Build history of the part. All positions in model axes, mm. A direction names the side the tool comes from. Round coordinates to 2 decimals unless told otherwise and drop trailing zeros. Loops run counter-clockwise (first coordinate to the right, second up) from the corner with the lowest first, then second, coordinate; pieces in that order, holes last. Notation, with made-up numbers: (-7.75, 63.5) - (44.25, 63.5) arc R19 ccw to (44.25, 84.5) - close; hole circle Ø8 at (59.5, 40). An arc over 180 degrees is marked (long way). Put each result on its own line as item: value. Start each with the question number.
from build123d import *

# Parameters (mm, degrees)
F1_DEPTH = 12


# Not quite as in the source:
# - a feature names something its author has since deleted; it is built from what else it names


with BuildPart() as f1:
    # F0 (on Front) → F1 (new body)
    with BuildSketch(Plane.XZ):
        with BuildLine():
            Line((-78.3512531443, 52.5226152241), (-78.3512531443, -23.4773847759))
            Line((-78.3512531443, -23.4773847759), (48.6487468557, -23.4773847759))
            Line((48.6487468557, -23.4773847759), (163.7198627451, -39.3522962011))
            ThreePointArc((163.7198627451, -39.3522962011), (169.4031778605, -34.3992082296), (163.7198627451, -29.4461202581))
            ThreePointArc((163.7198627451, -29.4461202581), (140.2372169997, 8.5604113595), (135.6487468557, 53))
            Line((135.6487468557, 53), (129.9201593475, 53))
            Line((129.9201593475, 53), (-55.8512531443, 53))
            Line((-55.8512531443, 53), (-78.3512531443, 53))
            Line((-78.3512531443, 53), (-78.3512531443, 52.5226152241))
        make_face()
        with BuildLine():
            Line((-63.3512531443, 7.5), (-63.3512531443, 21.5))
            Line((-63.3512531443, 21.5), (-63.3512531443, 35.5))
            ThreePointArc((-63.3512531443, 35.5), (-55.8512531443, 43), (-48.3512531443, 35.5))
            Line((-48.3512531443, 35.5), (-48.3512531443, 7.5))
            ThreePointArc((-48.3512531443, 7.5), (-55.8512531443, 0), (-63.3512531443, 7.5))
        make_face(mode=Mode.SUBTRACT)
        with BuildLine():
            Line((46.6487468557, 7.5), (46.6487468557, 21.5))
            Line((46.6487468557, 21.5), (46.6487468557, 35.5))
            ThreePointArc((46.6487468557, 35.5), (54.1487468557, 43), (61.6487468557, 35.5))
            Line((61.6487468557, 35.5), (61.6487468557, 7.5))
            ThreePointArc((61.6487468557, 7.5), (54.1487468557, 0), (46.6487468557, 7.5))
        make_face(mode=Mode.SUBTRACT)
    extrude(amount=F1_DEPTH)


solid = f1.part
1) Drill centre lines: line 1 (X direction, y = -9, z = 33); line 2 (X direction, y = -6.25, z = 20.5); line 3 (Z direction, x = 0.5, y = -3.25). Where is each one in solid material? Low to high. Write a range as [from, to].
2) Which spindle directions (+Z, -Z, +X, -X, +Y, -Y) get a long thin tool onto all of the face, cutting with end or side? Do faces 1 (the face through (140.442, -5.916, 7.964)), 2 (the face through (61.649, -6, 22)), 3 (the face through (-16, -6, -23.477)). Say none if no direction does.
3) Slice it at B-B, the plane x = -19.5. Write the cut outline in (y, z), and give its area (3 significant figures).
4) Drop flat-ended pins along their axis: pin 1 Ø3.5 at (y, z) = (-6, 25.5) entering from +X; pin 2 Ø6 at (y, z) = (-7, 19) entering from +X; pin 3 Ø1 at (y, z) = (-5, -22) entering from +X; pin 4 Ø6 at (x, z) = (102.5, 10.5) entering from +Y. Give the stop position or say it passes through.
5) Pull direction X, two halves, no side cores. Call faces 4 (the face through (-63.351, -6, 21)), 5 (the face through (105.379, -5.916, -31.304)), 6 (the face through (-56, -6, 43)), 7 (the face through (30, -6, 53)): pulls with the +X half, pulls with the -X half, needs draft (parallel to the pull), parting line crosses it, or undercut.
6) Slice it at A-A, the plane y = -9.25. Write the cut outline in (x, z), and give its area (3 significant figures).
Taken from the geometry:
1. line 1: x = [-78.35, -63.35], [-48.35, 46.65], [61.65, 135.2]
1. line 2: x = [-78.35, -63.35], [-48.35, 46.65], [61.65, 136.98]
1. line 3: z = [-23.48, 53]
2. face 1: +X, +Y, -Y
2. face 2: +Y, -Y
2. face 3: -Z, -X, +Y, -Y
3. outline: (-12, -23.48) - (0, -23.48) - (0, 53) - (-12, 53) - close
3. area: 918 mm2
4. pin 1: stops at x = 136.36
4. pin 2: stops at x = 138.02
4. pin 3: stops at x = 157.48
4. pin 4: stops at y = 0
5. face 4: undercut
5. face 5: pulls with the -X half
5. face 6: undercut
5. face 7: needs draft
6. outline: (-78.35, -23.48) - (48.65, -23.48) - (163.72, -39.35) arc R5 ccw (long way) to (163.72, -29.45) arc R100 cw to (135.65, 53) - (-78.35, 53) - close; hole (-63.35, 7.5) arc R7.5 ccw to (-48.35, 7.5) - (-48.35, 35.5) arc R7.5 ccw to (-63.35, 35.5) - close; hole (46.65, 7.5) arc R7.5 ccw to (61.65, 7.5) - (61.65, 35.5) arc R7.5 ccw to (46.65, 35.5) - close
6. area: 16,500 mm2
